The figure shows three views and two pictorial views of one solid part (mm, origin at its lowest corner). Answer the questions. Coordinates: 2 decimals unless noted, no trailing zeros. Loops run counter-clockwise (first coordinate to the right, second up) from the corner with the lowest first, then second, coordinate; pieces in that order, holes last. Notation, with made-up numbers: (44, 56.5) -> (57, 56.5) arc R14 cw to (57, 78.5) -> close; hole circle Ø11 at (-14.5, -13). An arc over 180 degrees is marked (long way). Answer in a Markdown table with one row per item.
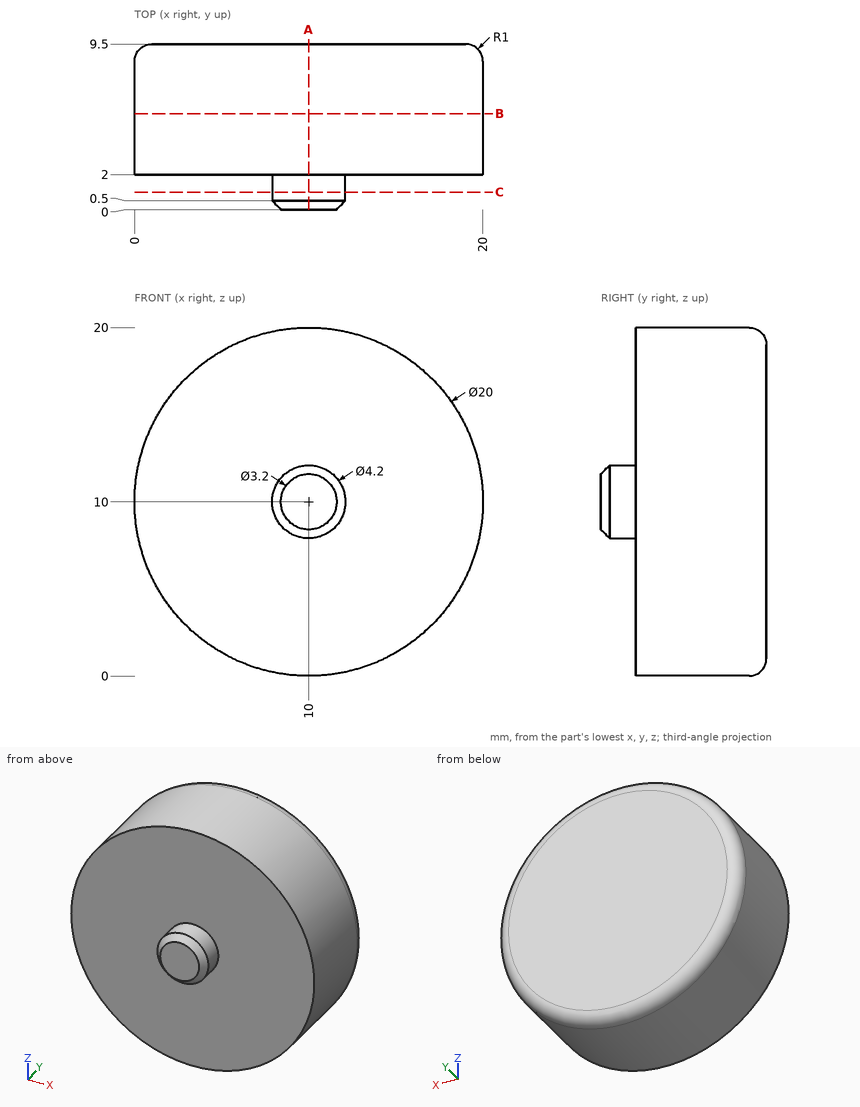
Item 1: Find the intervals of material crossed by probe 1 along Y at (x, z) = (7.25, 4.75); probe 2 along X at (y, z) = (5.75, 7.75); probe 3 along Z at (x, y) = (1.5, 2.25), in increasing order.
Findings below:
| item | result |
|---|---|
| probe 1 | y = 2 to 9.5 |
| probe 2 | x = 0.26 to 19.74 |
| probe 3 | z = 4.73 to 15.27 |
Item 2: A cutting plane is placed at A-A, the plane x = 10. Determine the outline of the cut face in (y, z), plus the area to 3 significant figures.
Findings below:
| item | result |
|---|---|
| outline | (0, 8.4) -> (0.5, 7.9) -> (2, 7.9) -> (2, 0) -> (8.5, 0) arc R1 ccw to (9.5, 1) -> (9.5, 19) arc R1 ccw to (8.5, 20) -> (2, 20) -> (2, 12.1) -> (0.5, 12.1) -> (0, 11.6) -> close |
| area | 158 mm2 |
Item 3: A cutting plane is placed at B-B, the plane y = 5.5. Determine the outline of the cut face in (x, z).
Findings below:
| item | result |
|---|---|
| outline | circle Ø20 at (10, 10) |
Item 4: A cutting plane is placed at C-C, the plane y = 1. Determine the outline of the cut face in (x, z), plus the area to 3 significant figures.
Findings below:
| item | result |
|---|---|
| outline | circle Ø4.2 at (10, 10) |
| area | 13.9 mm2 |
Item 5: Flat-ended cylindrical pins translate along their axes: pin 1 Ø2 at (x, y) = (7, 6.5) entering from -Z; pin 2 Ø2 at (y, z) = (4, 11.5) entering from -X; pin 3 Ø1 at (y, z) = (8.5, 7.5) entering from -X. Find the tip coordinate at first contact, or state that the pin passes through.
Findings below:
| item | result |
|---|---|
| pin 1 | stops at z = 0.2 |
| pin 2 | stops at x = 0.01 |
| pin 3 | stops at x = 0.2 |
